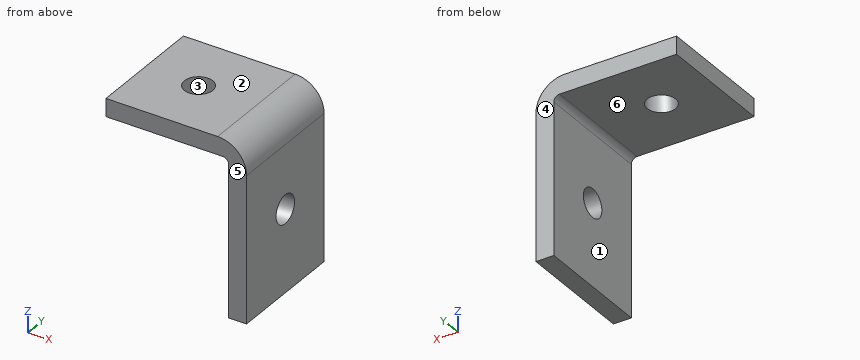
Autodesk Inventor part; units mm, degrees
ref_plane "YZ Plane" through (0, 0, 0) normal (1, 0, 0) x (0, 1, 0)
ref_plane "XZ Plane" through (0, 0, 0) normal (0, 1, 0) x (-1, 0, 0)
ref_plane "XY Plane" through (0, 0, 0) normal (0, 0, 1) x (1, 0, 0)
sketch "Sketch1" plane through (0, 0, 0) normal (0, 1, 0) x (-1, 0, 0)
  line L0 (0, 0) -> (12.16, 0)
  line L1 (12.16, 0) -> (12.16, -1.55)
  line L2 (1.55, -15.12) -> (0, -15.12)
  line L3 (0, -15.12) -> (0, 0)
  line L4 (10.61, -1.55) -> (1.55, -1.55)
  line L5 (1.55, -1.55) -> (1.55, -13.57)
  line L6 (10.61, -1.55) -> (12.16, -1.55)
  line L7 (1.55, -13.57) -> (1.55, -15.12)
  dimension "d2" = 1.55
  dimension "d3" = 12.16
  dimension "d4" = 15.12
extrude "Extrusion1" add sketch "Sketch1" along normal blind 10.3
sketch "Sketch2" plane through (-12.16, 0, 0) normal (0, 0, 1) x (1, 0, 0)
  line L0 (4.66, 14.5613) -> (4.66, -2.7265)
  line L1 (12.16, 0) -> (12.16, 10.3)
  line L2 (-7.6119, 5.15) -> (15.8963, 5.15)
  point P0 (12.16, 5.15)
  point P1 (4.66, 5.15)
  dimension "d7" = 7.5
hole "Hole1" at (-7.5, 5.15, 0) direction (0, 0, -1) diameter 2.459 end through all
sketch "Sketch3" plane through (0, 0, 0) normal (1, 0, 0) x (0, 0, -1)
  line L0 (-10.3606, 5.15) -> (23.1245, 5.15)
  line L1 (8, 14.2786) -> (8, -6.8061)
  line L2 (0, 0) -> (0, 10.3)
  point P0 (0, 5.15)
  point P1 (8, 5.15)
  dimension "d15" = 8
hole "Hole2" at (0, 5.15, -8) direction (-1, 0, 0) diameter 2.459 end through all
fillet "Fillet1" radius 2.5 1 edges at (0, 5.15, 0)
fillet "Fillet2" radius 0.5 1 edges at (-1.55, 5.15, -1.55)
properties part number "Threaded Right Support Farnell1466885"
Verification items for the finished model (mm, model axes). Face numbers are marked on the shaded views. A direction names the side the tool comes from. Give positions to 0.01 mm unless a question says otherwise; leave off trailing zeros. Loops run counter-clockwise (first coordinate to the right, second up) from the corner with the lowest first, then second, coordinate; pieces in that order, holes last.
1. Mould release check, pull along Y, two halves, no side actions. Record for the marked faces 3, 4, 5 and 6: released by +Y, released by -Y, zero draft, split by the parting line, or undercut.
2. Set-up check for the marked faces 1 and 2: record each of +Z, -Z, +X, -X, +Y, -Y from which the full face is reachable in a straight line by a thin tool's end or side.
3. Section check C-C, the plane y = 5.15. Enter the section's corners in (x, z).
4. Thickness scan on line 1 (Y direction, x = -0.95, z = -8); line 2 (Z direction, x = -9, y = 8.5). Record the ranges inside material, lowest first.
5. Section check B-B, the plane z = -8. Enter the section's corners in (x, y), then the cut area to 3 significant figures.
6. Section check D-D, the plane y = 2.25. Enter the section's corners in (x, z).
7. Section check A-A, the plane x = -7.5. Enter the section's corners in (y, z), then the cut area to 3 significant figures.
8. Go/stop test with flat-tipped pins: pin 1 Ø1 at (x, y) = (-8.5, 9) entering from -Z; pin 2 Ø3 at (x, y) = (-7.5, 5.15) entering from +Z; pin 3 Ø3 at (y, z) = (4.5, -11.5) entering from -X; pin 4 Ø1.5 at (y, z) = (5.15, -8) entering from +X. Record where each tip stops, or that it passes through.
Geometry says:
1. face 3: undercut
1. face 4: released by +Y
1. face 5: released by -Y
1. face 6: zero draft
2. face 1: -Z, -X, +Y, -Y
2. face 2: +Z, +X, -X, +Y, -Y
3. outline: (-12.16, -1.55) - (-8.73, -1.55) - (-8.73, 0) - (-12.16, 0) - close; (-6.27, -1.55) - (-2.05, -1.55) arc R0.5 cw to (-1.55, -2.05) - (-1.55, -6.77) - (0, -6.77) - (0, -2.5) arc R2.5 ccw to (-2.5, 0) - (-6.27, 0) - close; (-1.55, -15.12) - (0, -15.12) - (0, -9.23) - (-1.55, -9.23) - close
4. line 1: y = 0 to 3.92, 6.38 to 10.3
4. line 2: z = -1.55 to 0
5. outline: (-1.55, 0) - (0, 0) - (0, 3.92) - (-1.55, 3.92) - close; (-1.55, 6.38) - (0, 6.38) - (0, 10.3) - (-1.55, 10.3) - close
5. area: 12.2 mm2
6. outline: (-12.16, -1.55) - (-2.05, -1.55) arc R0.5 cw to (-1.55, -2.05) - (-1.55, -15.12) - (0, -15.12) - (0, -2.5) arc R2.5 ccw to (-2.5, 0) - (-12.16, 0) - close
7. outline: (0, -1.55) - (3.92, -1.55) - (3.92, 0) - (0, 0) - close; (6.38, -1.55) - (10.3, -1.55) - (10.3, 0) - (6.38, 0) - close
7. area: 12.2 mm2
8. pin 1: stops at z = -1.55
8. pin 2: stops at z = 0
8. pin 3: stops at x = -1.55
8. pin 4: passes through
